from build123d import *

# Parameters (mm, degrees)
SPLIT_CAP_WITH_RAISED_FLAT_WASHER_SEATS_DEPTH = 14
M4_THROUGH_HOLES_DEPTH                        = 60.969492244
M4_THROUGH_HOLES_DEPTH_BACK                   = 60.969492244
SKETCH2_R                                     = 2.25


with BuildPart() as part:
    # Split cap with raised flat washer se 2 → Split cap with raised flat washer seats (new body)
    with BuildSketch(Plane.XY):
        with BuildLine():
            Line((19.855477834, 37.5), (29.5, 37.5))
            Line((29.5, 37.5), (29.5, 28.8))
            Line((29.5, 28.8), (18.497567408, 28.8))
            ThreePointArc((18.497567408, 28.8), (0, 47), (-18.497567408, 28.8))
            Line((-18.497567408, 28.8), (-29.5, 28.8))
            Line((-29.5, 28.8), (-29.5, 37.5))
            Line((-29.5, 37.5), (-19.855477834, 37.5))
            ThreePointArc((-19.855477834, 37.5), (0, 50.3), (19.855477834, 37.5))
        make_face()
    extrude(amount=SPLIT_CAP_WITH_RAISED_FLAT_WASHER_SEATS_DEPTH)

    # Sketch2 → M4 through holes (cut, two sides: drawn at the far end of the back side and taken through both)
    with BuildSketch(Plane(origin=(0, 0, 0), x_dir=(1, 0, 0), z_dir=(0, 1, 0)).offset(-M4_THROUGH_HOLES_DEPTH_BACK)):
        with Locations(Location((-24.5, -7, 0), (0, 0, 90))):
            Circle(SKETCH2_R)
        with Locations(Location((24.5, -7, 0), (0, 0, 90))):
            Circle(SKETCH2_R)
    extrude(amount=M4_THROUGH_HOLES_DEPTH + M4_THROUGH_HOLES_DEPTH_BACK, mode=Mode.SUBTRACT)


solid = part.part
Design review of the part built by this model. Coordinates are the model's own, in mm. A direction names the side the tool comes from. Give positions to 0.01 mm unless a question says otherwise; leave off trailing zeros. Write each loop counter-clockwise with the first axis right and the second up, starting at its lowest first coordinate (ties: lowest second). Pieces come first, ordered by that corner, then holes. Notation, with made-up numbers: M 52,-37 L 105,-37 A18 ccw 105,-7 Z; hole C 22,26.25 d4. An arc over 180 degrees is marked long. Answer as a JSON object with one key per item and string values. Group by question number.
1) Tool access review of faces 1 (the face through (-27, 37.5, 7)), 2 (the face through (-22.304, 33.089, 7.488)), 3 (the face through (27, 37.5, 7)): name each direction out of +Z, -Z, +X, -X, +Y, -Y from which nothing blocks a thin tool from reaching the whole face with its end or side.
2) For line 1 along X through (y, z) = (34.25, 7.25); line 2 along X through (y, z) = (33.75, 7); line 3 along Y through (x, z) = (-24.5, 3), list the stretches that pass through material, from the lowest coordinate up.
3) We need section C-C (x = -24.5). Give the boundary of the cut face in (y, z), and give its area (4 significant figures).
4) Clearance check with flat-ended pins moving along their axes: pin 1 Ø7.5 at (x, z) = (26, 5.5) entering from +Y; pin 2 Ø8 at (x, z) = (-14.5, 10) entering from +Y; pin 3 Ø2 at (x, z) = (-5.5, 9) entering from +Y. State where each tip first meets the part, or that it passes through.
5) Mouldability with a two-part tool opening along X and no side actions: class faces 4 (the face through (-0.35, 50.297, 6.902)), 5 (the face through (0, 47, 7)), 6 (the face through (0, 48, 14)) as released by +X, released by -X, zero draft, split by the parting line, or undercut.
6) We need section D-D (y = 40.5). Give the boundary of the cut face in (x, z).
7) We need section A-A (y = 34.5). Give the boundary of the cut face in (x, z).
Answer key:
{
 "1": {"face 1": "+Z, -Z, -X, +Y", "face 2": "+Y, -Y", "face 3": "+Z, -Z, +X, +Y"},
 "2": {"line 1": "x = -29.5 to -26.74, -22.26 to -17.58, 17.58 to 22.26, 26.74 to 29.5", "line 2": "x = -29.5 to -26.75, -22.25 to -17.74, 17.74 to 22.25, 26.75 to 29.5", "line 3": "y = 28.8 to 37.5"},
 "3": {"outline": "M 28.8,0 L 37.5,0 L 37.5,4.75 L 28.8,4.75 Z; M 28.8,9.25 L 37.5,9.25 L 37.5,14 L 28.8,14 Z", "area": "82.65 mm²"},
 "4": {"pin 1": "stops at y = 37.5", "pin 2": "stops at y = 47.6", "pin 3": "stops at y = 49.83"},
 "5": {"face 4": "split by the parting line", "face 5": "undercut", "face 6": "zero draft"},
 "6": {"outline": "M -18.2,0 L -14.08,0 L -14.08,14 L -18.2,14 Z; M 14.08,0 L 18.2,0 L 18.2,14 L 14.08,14 Z"},
 "7": {"outline": "M -29.5,0 L -17.5,0 L -17.5,14 L -29.5,14 Z; M 17.5,0 L 29.5,0 L 29.5,14 L 17.5,14 Z; hole C -24.5,7 d4.5; hole C 24.5,7 d4.5"}
}
